Input: part model. Units: mm. Frame: model coordinates. A direction names the side the tool comes from. Coordinates: 2 decimals unless noted, no trailing zeros. Order: outer loops, then holes, each group sorted by start corner. A loop starts at its lowest first (then second) coordinate and runs counter-clockwise, first axis right, second up. Notation, with made-up numbers: (75.25, 29) -> (86.25, 29) arc R16 cw to (86.25, 60) -> close; hole circle Ø10 at (-17.75, 59.5). An arc over 180 degrees is marked (long way). Answer as CSV lines item,"result".
from build123d import *

# Parameters (mm, degrees)
SKETCH1_R           = 3.175
BOSS_EXTRUDE1_DEPTH = 12.7
CUT_SWEEP1_PITCH    = 1.27
SKETCH4_OUTSIDE_W   = 14
SKETCH4_OUTSIDE_H   = 14
SKETCH4_OUTSIDE_R   = 2.21262927
CUT_EXTRUDE1_DEPTH  = 1.27
CUT_EXTRUDE1_DRAFT  = -45
CUT_EXTRUDE2_DEPTH  = 2.38125
BOSS_EXTRUDE2_START = -6.35
SKETCH8_R           = 3.175
BOSS_EXTRUDE2_DEPTH = 2.3876
SKETCH9_R           = 3.5687
SKETCH9_R_2         = 3.175
BOSS_EXTRUDE3_DEPTH = 0.762


with BuildPart() as part:
    # Sketch1 → Boss-Extrude1 (new body)
    with BuildSketch(Plane(origin=(0, 0, 0), x_dir=(1, 0, 0), z_dir=(0, 1, 0))):
        with Locations(Location((-12.7, 0, 0), (0, 0, 270))):
            Circle(SKETCH1_R)
    extrude(amount=-BOSS_EXTRUDE1_DEPTH)

    # Cut-Sweep1: the profile of Sketch3 screwed along a right-hand helix of 11 turns, 8 arcs to a turn; built about Z, then put on its axis
    cut_sweep1_z = Axis((0, 0, 0), (0, 0, 1))
    cut_sweep1_corners = [(2.350110803, 0, -0.47625), (3.243740766, 0, 0.0396875), (3.243740766, 0, -1.1509375), (2.350110803, 0, -0.635)]
    with BuildLine(mode=Mode.PRIVATE) as cut_sweep1_profile:
        Line(cut_sweep1_corners[0], cut_sweep1_corners[1])
        Line(cut_sweep1_corners[1], cut_sweep1_corners[2])
        Line(cut_sweep1_corners[2], cut_sweep1_corners[3])
        Line(cut_sweep1_corners[3], cut_sweep1_corners[0])
    cut_sweep1_cap = Face(cut_sweep1_profile.wire())
    cut_sweep1_turn_angles = [0, 22.5, 45, 67.5, 90, 112.5, 135, 157.5, 180, 202.5, 225, 247.5, 270, 292.5, 315, 337.5, 360]
    cut_sweep1_turn_weights = [1, 0.9238795325112867, 1, 0.9238795325112867, 1, 0.9238795325112867, 1, 0.9238795325112867, 1, 0.9238795325112867, 1, 0.9238795325112867, 1, 0.9238795325112867, 1, 0.9238795325112867, 1]
    cut_sweep1_turn_rails = [Edge.make_bspline([Vector(p[0], p[1], 0).rotate(cut_sweep1_z, cut_sweep1_turn_angles[k]) / cut_sweep1_turn_weights[k] + Vector(0, 0, p[2] + CUT_SWEEP1_PITCH * cut_sweep1_turn_angles[k] / 360) for k in range(17)], [0, 0, 0, 1, 1, 2, 2, 3, 3, 4, 4, 5, 5, 6, 6, 7, 7, 8, 8, 8], 2, cut_sweep1_turn_weights) for p in cut_sweep1_corners]
    cut_sweep1_turn_sides = [Face.make_surface_from_curves(cut_sweep1_turn_rails[p[0]], cut_sweep1_turn_rails[p[1]]) for p in [(0, 1), (1, 2), (2, 3), (3, 0)]]
    cut_sweep1 = Plane(origin=(-12.7, -12.7, 0), x_dir=(0, 0, -1), z_dir=(0, 1, 0)) * Solid(Shell([*[p.moved(Location((0, 0, CUT_SWEEP1_PITCH * i))) for i in range(11) for p in cut_sweep1_turn_sides], cut_sweep1_cap, cut_sweep1_cap.rotate(cut_sweep1_z, 3960).moved(Location((0, 0, CUT_SWEEP1_PITCH * 3960 / 360)))]))
    add(cut_sweep1, mode=Mode.SUBTRACT)


with BuildPart() as cut_extrude1_tool:
    # Sketch4 outside → Cut-Extrude1 (with draft: the straight prism first)
    with BuildSketch(Plane.XZ.offset(12.7)):
        with Locations((-12.7, 0)):
            Rectangle(SKETCH4_OUTSIDE_W, SKETCH4_OUTSIDE_H)
        with Locations((-12.7, 0)):
            Circle(SKETCH4_OUTSIDE_R, mode=Mode.SUBTRACT)
    extrude(amount=-CUT_EXTRUDE1_DEPTH)
    # Cut-Extrude1: the draft: its side faces are tilted about the plane it starts from
    cut_extrude1_sides = [cut_extrude1_tool.faces().sort_by_distance(p)[0] for p in [
        (-12.7, -12.065, -7),
        (-5.7, -12.065, 0),
        (-12.7, -12.065, 7),
        (-19.7, -12.065, 0),
        (-14.91262927, -12.065, 0),
    ]]
    draft(cut_extrude1_sides, Plane.XZ.offset(12.7), CUT_EXTRUDE1_DRAFT)


with BuildPart() as part_1:
    add(part.part)

    # Cut-Extrude1: cut by cut_extrude1_tool
    add(cut_extrude1_tool.part, mode=Mode.SUBTRACT)

    # Sketch5 → Revolve1 (revolve)
    with BuildSketch(Plane.XY, mode=Mode.PRIVATE) as revolve1_sk:
        with BuildLine():
            Line((-12.7, 0), (-12.7, 3.3528))
            Line((-12.7, 3.3528), (-15.875, 3.3528))
            ThreePointArc((-15.875, 3.3528), (-17.240019085, 2.263204136), (-18.2499, 0.8382))
            Line((-18.2499, 0.8382), (-19.6342, 0.8382))
            Line((-19.6342, 0.8382), (-19.6342, 0))
            Line((-19.6342, 0), (-12.7, 0))
        make_face()
    revolve(revolve1_sk.sketch.rotate(Axis((-12.7, 0, 0), (0, 1, 0)), 270), axis=Axis((-12.7, 0, 0), (0, 1, 0)))

    # Sketch6 → Cut-Extrude2 (cut)
    with BuildSketch(Plane(origin=(0, 3.3528, 0), x_dir=(1, 0, 0), z_dir=(0, 1, 0))):
        Polygon((-12.7, 2.291358881), (-14.684375, 1.14567944), (-14.684375, -1.14567944), (-12.7, -2.291358881), (-10.715625, -1.14567944), (-10.715625, 1.14567944), align=None)
    extrude(amount=-CUT_EXTRUDE2_DEPTH, mode=Mode.SUBTRACT)

    # Cut-Extrude3 cone 1 section (through the dimple's axis) → Cut-Extrude3 (revolve, cut)
    with BuildSketch(Plane(origin=(-12.7, 3.3528, 0), x_dir=(0, 0, 1), z_dir=(1, 0, 0))):
        Polygon((0, 0), (2.291358881, 0), (0, 2.291358881), align=None)
    revolve(axis=Axis((-12.7, 3.3528, 0), (0, -1, 0)), mode=Mode.SUBTRACT)


with BuildPart() as body_2:
    # Body-Move/Copy1: copy of part
    add(part_1.part.moved(Location((25.4, 0, 0))))


with BuildPart() as body_3:
    # Sketch8 → Boss-Extrude2 (new body)
    with BuildSketch(Plane(origin=(0, 0, 0), x_dir=(1, 0, 0), z_dir=(0, 1, 0)).offset(BOSS_EXTRUDE2_START)):
        with BuildLine():
            Line((-21.474187891, 5.6261), (21.474187891, 5.6261))
            ThreePointArc((21.474187891, 5.6261), (23.8125, 0), (21.474187891, -5.6261))
            Line((21.474187891, -5.6261), (-21.474187891, -5.6261))
            ThreePointArc((-21.474187891, -5.6261), (-23.8125, 0), (-21.474187891, 5.6261))
        make_face()
        with Locations(Location((-12.7, 0, 0), (0, 0, 270))):
            Circle(SKETCH8_R, mode=Mode.SUBTRACT)
        with Locations(Location((12.7, 0, 0), (0, 0, 270))):
            Circle(SKETCH8_R, mode=Mode.SUBTRACT)
    extrude(amount=-BOSS_EXTRUDE2_DEPTH)

    # Sketch9 → Boss-Extrude3 (add)
    # profile 1 of 2: a face of its own
    with BuildSketch(Plane.XZ.offset(8.7376)):
        with Locations(Location((-12.7, 0, 0), (0, 0, 90))):
            Circle(SKETCH9_R)
        with Locations(Location((-12.7, 0, 0), (0, 0, 90))):
            Circle(SKETCH9_R_2, mode=Mode.SUBTRACT)
    # profile 2 of 2: a face of its own
    with BuildSketch(Plane.XZ.offset(8.7376)):
        with Locations(Location((12.7, 0, 0), (0, 0, 90))):
            Circle(SKETCH9_R)
        with Locations(Location((12.7, 0, 0), (0, 0, 90))):
            Circle(SKETCH9_R_2, mode=Mode.SUBTRACT)
    extrude(amount=BOSS_EXTRUDE3_DEPTH)


solid = body_3.part
1. Cut plane B-B (x = -14.5). Return the cut outline in (y, z).
Findings:
outline,"(-9.5, -3.08) -> (-8.74, -3.08) -> (-8.74, -5.63) -> (-6.35, -5.63) -> (-6.35, -2.62) -> (-9.5, -2.62) -> close; (-9.5, 2.62) -> (-6.35, 2.62) -> (-6.35, 5.63) -> (-8.74, 5.63) -> (-8.74, 3.08) -> (-9.5, 3.08) -> close"
2. Cut plane D-D (x = 12.7). Return the cut outline in (y, z) (3 decimals).
Findings:
outline,"(-9.5, -3.569) -> (-8.738, -3.569) -> (-8.738, -5.626) -> (-6.35, -5.626) -> (-6.35, -3.175) -> (-9.5, -3.175) -> close; (-9.5, 3.175) -> (-6.35, 3.175) -> (-6.35, 5.626) -> (-8.738, 5.626) -> (-8.738, 3.569) -> (-9.5, 3.569) -> close"
3. Mould query, pull axis X, two halves, no side actions, for faces 3 (the face through (0, -8, -5.626)), 4 (the face through (-23.81, -7.53, 0.09)), 5 (the face through (0, -8.738, 0)). Classes: released by +X, released by -X, zero draft, split by the parting line, or undercut.
Findings:
face 3,"zero draft"
face 4,"released by -X"
face 5,"undercut"
4. Ray query, line 1 along X through (y, z) = (-9.15, 0) (3 decimals); line 2 along X through (y, z) = (-6.95, 0) (1 decimal); line 3 along Z through (x, y) = (-12.7, -9.1) (3 decimals). Return the intervals inside material, ascending.
Findings:
line 1,"x = -16.269 to -15.875, -9.525 to -9.131, 9.131 to 9.525, 15.875 to 16.269"
line 2,"x = -23.8 to -15.9, -9.5 to 9.5, 15.9 to 23.8"
line 3,"z = -3.569 to -3.175, 3.175 to 3.569"
5. Cut plane A-A (z = 0). State how many separate pieces and enclosed holes the cut face has, plus the area to 3 significant figures.
Findings:
separate pieces,"3"
enclosed holes,"0"
area,"84.6 mm2"
6. Reachability of faces 1 (the face through (0, -6.35, 0)), 2 (the face through (9.16, -9.11, -0.46)) from +Z, -Z, +X, -X, +Y, -Y: full face, straight path, thin tool, end or side. Return the list, or none.
Findings:
face 1,"+Z, -Z, +X, -X, +Y"
face 2,"-Y"
7. Contact query for flat-ended pins moving along their axis: pin 1 (3 mm diameter, centred on x = -1, z = -2, fed in from -Y); pin 2 (1.5 mm diameter, centred on x = -9.5, z = 2, fed in from -Y). Output: stop coordinate, or through.
Findings:
pin 1,"stops at y = -8.74"
pin 2,"stops at y = -9.5"
